For this review, use the dimensioned drawing (mm, ordinates from the lowest corner) and the shaded views. Give positions to 0.01 mm unless a question says otherwise; leave off trailing zeros. Order: outer loops, then holes, each group sorted by start corner. A loop starts at its lowest first (then second) coordinate and runs counter-clockwise, first axis right, second up. Notation, with made-up numbers: (41, 63.5) - (79, 63.5) arc R20 cw to (79, 89.5) - close; hole circle Ø9 at (-20, 79.5). An arc over 180 degrees is marked (long way). One line per item, written item: value.
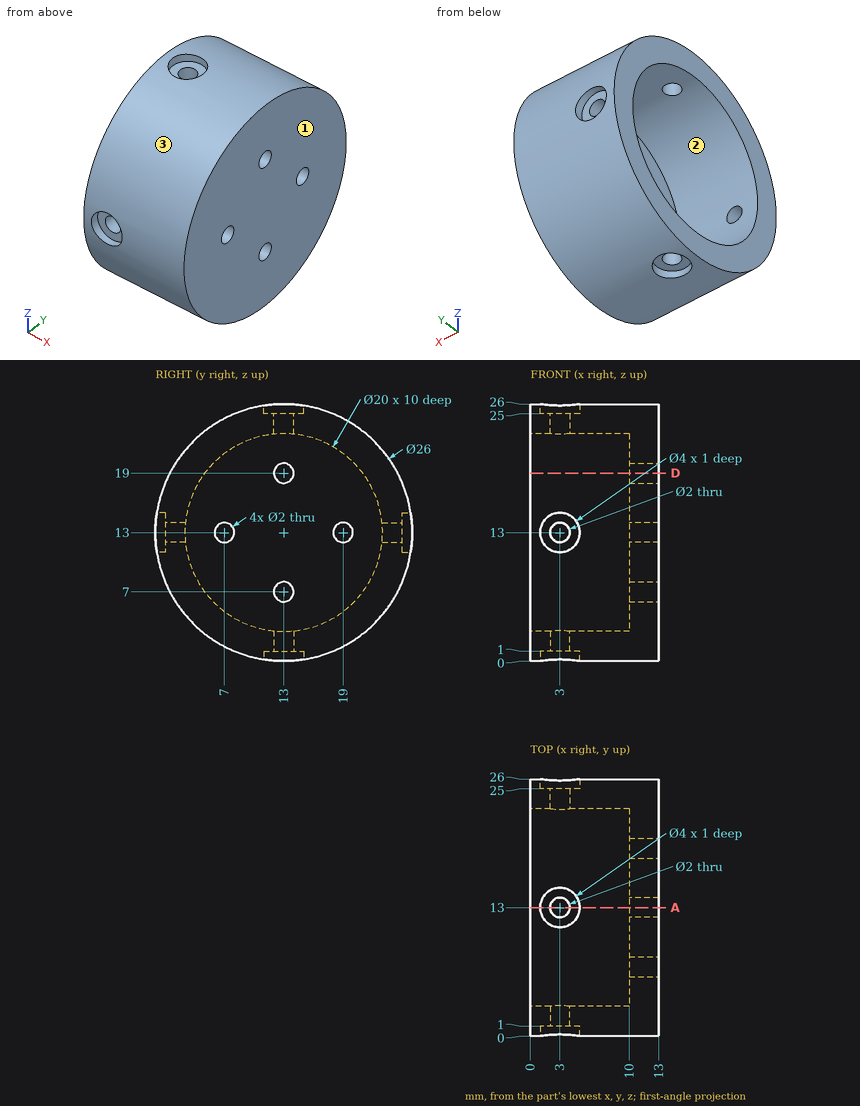
(1) Draft analysis for pull direction Z (two halves, no side actions). For the marked faces 1, 2 and 3, state which applies: pulls with the +Z half, pulls with the -Z half, needs draft (parallel to the pull), parting line crosses it, or undercut.
Answers below:
face 1: needs draft
face 2: undercut
face 3: parting line crosses it
(2) Take a section at D-D (z = 19). Write out the cut boundary in (x, y).
Answers below:
outline: (0, 1.47) - (13, 1.47) - (13, 12) - (10, 12) - (10, 5) - (0, 5) - close; (0, 21) - (10, 21) - (10, 14) - (13, 14) - (13, 24.53) - (0, 24.53) - close
(3) Wall thickness on line 1 (Z direction, x = 10.6, y = 13); line 2 (X direction, y = 6, z = 17.25); line 3 (Z direction, x = 1, y = 11): over which ranges is each line inside the solid? List them lowest first. Write a range as from..to.
Answers below:
line 1: z = 0..6, 8..18, 20..26
line 2: x = 10..13
line 3: z = 0.15..3.2, 22.8..25.85
(4) Take a section at A-A (y = 13). Give the number of separate pieces and of enclosed holes in the cut face, then the cut area to 3 significant figures.
Answers below:
separate pieces: 5
enclosed holes: 0
area: 110 mm^2
(5) For P1, Ø3, axis at x = 3, y = 13, coming from the +Z side; P2, Ø3.5, axis at x = 3, z = 13, coming from the -Y side; P3, Ø4, axis at x = 8, y = 7.5, coming from the +Z side, all flat-tipped, find the tip position at first contact; note any pin that passes through.
Answers below:
P1: stops at z = 25
P2: stops at y = 1
P3: stops at z = 25.52
